```python
from build123d import *

# Parameters (mm, degrees)
F1_DEPTH = 25.4
F2_DEPTH = 1.27
F3_W     = 8.89
F3_H     = 21.59
F4_DEPTH = 25.4


with BuildPart() as f1:
    # F0 (on Top) → F1 (new body)
    with BuildSketch(Plane.XY):
        with BuildLine():
            Line((59.960537, 45.825542), (-49.74861, 45.825542))
            ThreePointArc((-49.74861, 45.825542), (-60.884126, 41.21306), (-65.496609, 30.077543))
            Line((-65.496609, 30.077543), (-65.496609, -29.551196))
            Line((-65.496609, -29.551196), (44.212538, -29.551196))
            ThreePointArc((44.212538, -29.551196), (55.348055, -24.938714), (59.960537, -13.803197))
            Line((59.960537, -13.803197), (59.960537, 45.825542))
        make_face()
        with BuildLine():
            ThreePointArc((-63.71861, 30.077543), (-59.626891, 39.955824), (-49.74861, 44.047543))
            Line((-49.74861, 44.047543), (-40.670957, 44.047543))
            Line((-40.670957, 44.047543), (-40.670957, -27.773197))
            Line((-40.670957, -27.773197), (-63.71861, -27.773197))
            Line((-63.71861, -27.773197), (-63.71861, 30.077543))
        make_face(mode=Mode.SUBTRACT)
        with BuildLine():
            Line((-39.400957, 44.047543), (58.182538, 44.047543))
            Line((58.182538, 44.047543), (58.182538, 33.949472))
            Line((58.182538, 33.949472), (17.172182, 33.949472))
            Line((17.172182, 33.949472), (17.172182, 32.679472))
            Line((17.172182, 32.679472), (58.182538, 32.679472))
            Line((58.182538, 32.679472), (58.182538, -13.803197))
            ThreePointArc((58.182538, -13.803197), (54.090819, -23.681479), (44.212538, -27.773197))
            Line((44.212538, -27.773197), (-39.400957, -27.773197))
            Line((-39.400957, -27.773197), (-39.400957, 32.679472))
            Line((-39.400957, 32.679472), (0, 32.679472))
            Line((0, 32.679472), (0, 33.949472))
            Line((0, 33.949472), (-39.400957, 33.949472))
            Line((-39.400957, 33.949472), (-39.400957, 44.047543))
        make_face(mode=Mode.SUBTRACT)
    extrude(amount=F1_DEPTH)

    # F0 (on Top) → F2 (join)
    with BuildSketch(Plane.XY):
        with BuildLine():
            Line((-40.670957, 44.047543), (-49.74861, 44.047543))
            ThreePointArc((-49.74861, 44.047543), (-59.626891, 39.955824), (-63.71861, 30.077543))
            Line((-63.71861, 30.077543), (-63.71861, -27.773197))
            Line((-63.71861, -27.773197), (-40.670957, -27.773197))
            Line((-40.670957, -27.773197), (-40.670957, 44.047543))
        make_face()
        with BuildLine():
            Line((58.182538, 33.949472), (58.182538, 44.047543))
            Line((58.182538, 44.047543), (-39.400957, 44.047543))
            Line((-39.400957, 44.047543), (-39.400957, 33.949472))
            Line((-39.400957, 33.949472), (0, 33.949472))
            Line((0, 33.949472), (0, 32.679472))
            Line((0, 32.679472), (-39.400957, 32.679472))
            Line((-39.400957, 32.679472), (-39.400957, -27.773197))
            Line((-39.400957, -27.773197), (44.212538, -27.773197))
            ThreePointArc((44.212538, -27.773197), (54.090819, -23.681479), (58.182538, -13.803197))
            Line((58.182538, -13.803197), (58.182538, 32.679472))
            Line((58.182538, 32.679472), (17.172182, 32.679472))
            Line((17.172182, 32.679472), (17.172182, 33.949472))
            Line((17.172182, 33.949472), (58.182538, 33.949472))
        make_face()
    extrude(amount=F2_DEPTH)

    # F3 (on face) → F4 (cut)
    with BuildSketch(Plane.XZ.offset(29.551196)):
        with Locations((-40.575533, 12.065)):
            Rectangle(F3_W, F3_H)
    extrude(amount=-F4_DEPTH, mode=Mode.SUBTRACT)


solid = f1.part
```
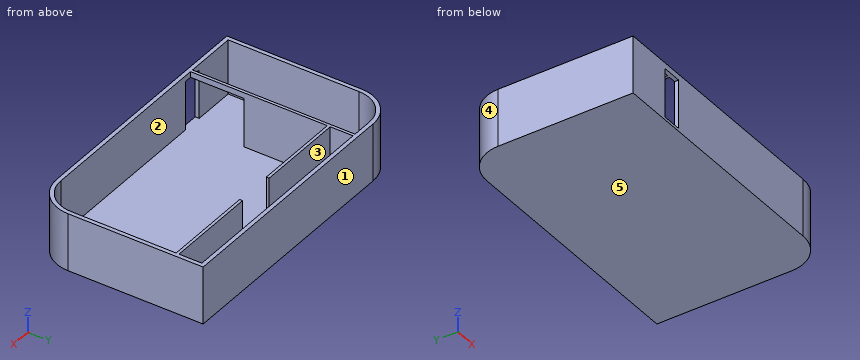
Model file for the job. Use its own axes, mm. Face numbers are marked on the shaded views. A direction names the side the tool comes from. Coordinates: 2 decimals unless noted, no trailing zeros. Order: outer loops, then holes, each group sorted by start corner. A loop starts at its lowest first (then second) coordinate and runs counter-clockwise, first axis right, second up. Notation, with made-up numbers: (-17.5, 76) -> (16.5, 76) arc R19 cw to (16.5, 83) -> close; hole circle Ø10 at (-33.5, 40). An arc over 180 degrees is marked (long way). Return JSON: item names as keys, results as strings.
Item 1: Slice it at A-A (x = 15). Write the cut outline in (y, z), then the cut area to 3 significant figures.
Model answer:
{"outline": "(-29.55, 0) -> (45.83, 0) -> (45.83, 25.4) -> (44.05, 25.4) -> (44.05, 1.27) -> (-27.77, 1.27) -> (-27.77, 25.4) -> (-29.55, 25.4) -> close", "area": "182 mm²"}
Item 2: Mould opens along X. For the marked faces 3, 4 and 5 say: pulls with the +X half, pulls with the -X half, needs draft (parallel to the pull), parting line crosses it, or undercut.
Model answer:
{"face 3": "undercut", "face 4": "pulls with the -X half", "face 5": "needs draft"}
Item 3: Slice it at D-D (y = 22.5). Write the cut outline in (x, z), then the cut area to 3 significant figures.
Model answer:
{"outline": "(-65.5, 0) -> (59.96, 0) -> (59.96, 25.4) -> (58.18, 25.4) -> (58.18, 1.27) -> (-39.4, 1.27) -> (-39.4, 25.4) -> (-40.67, 25.4) -> (-40.67, 1.27) -> (-63.72, 1.27) -> (-63.72, 25.4) -> (-65.5, 25.4) -> close", "area": "276 mm²"}
Item 4: Slice it at C-C (z = 9.5). Write the cut outline in (x, y), then the cut area to 3 significant figures.
Model answer:
{"outline": "(-65.5, -29.55) -> (-45.02, -29.55) -> (-45.02, -27.77) -> (-63.72, -27.77) -> (-63.72, 30.08) arc R13.97 cw to (-49.75, 44.05) -> (-40.67, 44.05) -> (-40.67, -4.15) -> (-39.4, -4.15) -> (-39.4, 32.68) -> (0, 32.68) -> (0, 33.95) -> (-39.4, 33.95) -> (-39.4, 44.05) -> (58.18, 44.05) -> (58.18, 33.95) -> (17.17, 33.95) -> (17.17, 32.68) -> (58.18, 32.68) -> (58.18, -13.8) arc R13.97 cw to (44.21, -27.77) -> (-36.13, -27.77) -> (-36.13, -29.55) -> (44.21, -29.55) arc R15.75 ccw to (59.96, -13.8) -> (59.96, 45.83) -> (-49.75, 45.83) arc R15.75 ccw to (-65.5, 30.08) -> close", "area": "826 mm²"}
Item 5: Slice it at B-B (y = -7). Write the cut outline in (x, z), then the cut area to 3 significant figures.
Model answer:
{"outline": "(-65.5, 0) -> (59.96, 0) -> (59.96, 25.4) -> (58.18, 25.4) -> (58.18, 1.27) -> (-63.72, 1.27) -> (-63.72, 25.4) -> (-65.5, 25.4) -> close; (-40.67, 22.86) -> (-39.4, 22.86) -> (-39.4, 25.4) -> (-40.67, 25.4) -> close", "area": "248 mm²"}
Item 6: 3-axis set-ups, long thin cutter, end or side, ignore diameter. For the marked faces 1 and 2: which of +Z, -Z, +X, -X, +Y, -Y reach the whole face in a straight line?
Model answer:
{"face 1": "+Z, -Z, +X, -X, +Y", "face 2": "+Z"}
Item 7: Wall check: line 1 along Y through (x, z) = (-30.5, 22.5); line 2 along X through (y, z) = (18.5, 13.5); line 3 along X through (y, z) = (37.5, 24.5). Give the ranges that are in metal, low to high. Write a range as from..to.
Model answer:
{"line 1": "y = -29.55..-27.77, 32.68..33.95, 44.05..45.83", "line 2": "x = -65.5..-63.72, -40.67..-39.4, 58.18..59.96", "line 3": "x = -63.64..-61.58, -40.67..-39.4, 58.18..59.96"}
Item 8: Pin check, flat tip, straight feed: P1, Ø3, axis at y = 40.5, z = 12.5, coming from the -X side. Stop position of the tip, or through.
Model answer:
{"P1": "stops at x = -62.73"}
